Input: part model. Units: mm. Frame: model coordinates. Face numbers are marked on the shaded views. A direction names the side the tool comes from. Coordinates: 2 decimals unless noted, no trailing zeros. Write each loop counter-clockwise with the first axis right and the second up, starting at its lowest first coordinate (ties: lowest second). Pieces come first, ordered by that corner, then holes. Notation, with made-up numbers: (-7, 48) - (4, 48) arc R16 ccw to (4, 76) - close; hole circle Ø7 at (24, 87). An arc over 180 degrees is marked (long way). Use CSV: the item, a comma, the result in double quotes.
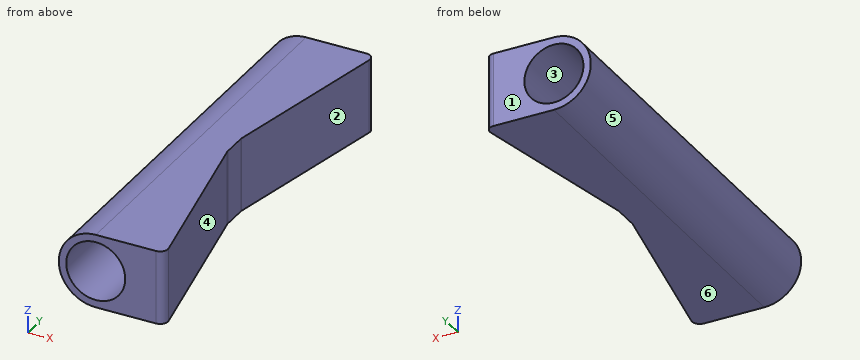
```python
from build123d import *

# Parameters (mm, degrees)
SKETCH1_R           = 14.2875
SKETCH1_R_2         = 11.4125
BOSS_EXTRUDE1_DEPTH = 152.4
SKETCH2_W           = 28.575
SKETCH2_H           = 152.4
BOSS_EXTRUDE2_DEPTH = 12.7
BOSS_EXTRUDE3_DEPTH = 152.4
CUT_EXTRUDE1_DEPTH  = 29.575
FILLET1_R           = 3


with BuildPart() as part:
    # Sketch1 → Boss-Extrude1 (new body)
    with BuildSketch(Plane(origin=(0, 0, 0), x_dir=(1, 0, 0), z_dir=(0, 1, 0))):
        Circle(SKETCH1_R)
        Circle(SKETCH1_R_2, mode=Mode.SUBTRACT)
    extrude(amount=BOSS_EXTRUDE1_DEPTH)



with BuildPart() as body_2:
    # Sketch2 → Boss-Extrude2 (new body)
    with BuildSketch(Plane(origin=(14.2875, 0, 0), x_dir=(0, 0, -1), z_dir=(1, 0, 0))):
        with Locations((0, 76.2)):
            Rectangle(SKETCH2_W, SKETCH2_H)
    extrude(amount=BOSS_EXTRUDE2_DEPTH)


with BuildPart() as part_1:
    add(part.part)

    add(body_2.part)  # Boss-Extrude3 merges body 2
    # Sketch3 → Boss-Extrude3 (add, through all)
    with BuildSketch(Plane(origin=(0, 152.4, 0), x_dir=(1, 0, 0), z_dir=(0, 1, 0))):
        with BuildLine():
            Line((14.2875, -14.2875), (0, -14.2875))
            ThreePointArc((0, -14.2875), (14.2875, 0), (0, 14.2875))
            Line((0, 14.2875), (14.2875, 14.2875))
            Line((14.2875, 14.2875), (26.9875, 14.2875))
            Line((26.9875, 14.2875), (26.9875, -14.2875))
            Line((26.9875, -14.2875), (14.2875, -14.2875))
        make_face()
    extrude(amount=-BOSS_EXTRUDE3_DEPTH)

    # Sketch5 → Cut-Extrude1 (cut, through all)
    with BuildSketch(Plane.XY.offset(14.2875)):
        Polygon((26.9875, 0), (12.897222949, 71.2), (12.897222949, 81.2), (26.9875, 152.4), align=None)
    extrude(amount=-CUT_EXTRUDE1_DEPTH, mode=Mode.SUBTRACT)

    # Fillet1
    fillet1_edges = [part_1.edges().sort_by_distance(p)[0] for p in [
        (26.9875, 0, 0),
        (26.9875, 152.4, 0),
        (12.897222949, 71.2, 0),
        (12.897222949, 81.2, 0),
    ]]
    fillet(fillet1_edges, radius=FILLET1_R)


solid = part_1.part
```
(1) Reachability of the marked faces 1 and 2 from +Z, -Z, +X, -X, +Y, -Y: full face, straight path, thin tool, end or side. Return the list, or none.
Check values:
face 1,"+Z, -Z, +X, -X, +Y"
face 2,"+Z, -Z, +X"
(2) Cut plane C-C on y = 35. Return loops of the section in (x, z) (1 decimal), and give its area (3 significant figures).
Check values:
outline,"(0, -14.3) - (20.1, -14.3) - (20.1, 14.3) - (0, 14.3) arc R14.3 ccw to start; hole circle Ø22.8 at (0, 0)"
area,"485 mm^2"
(3) Cut plane A-A on z = 0. Return loops of the section in (x, y).
Check values:
outline,"(-14.29, 0) - (-11.41, 0) - (-11.41, 152.4) - (-14.29, 152.4) - close; (11.41, 0) - (23.34, 0) arc R3 ccw to (26.28, 3.58) - (12.95, 70.91) arc R3 cw to (12.9, 71.49) - (12.9, 80.91) arc R3 cw to (12.95, 81.49) - (26.28, 148.82) arc R3 ccw to (23.34, 152.4) - (11.41, 152.4) - close"
(4) Ray query, probe 1 along X at (y, z) = (80, 0.25); probe 2 along X at (y, z) = (7, -0.25); probe 3 along Z at (x, y) = (-9, 126.5). Return the intervals inside material, ascending. Write a range as from..to.
Check values:
probe 1,"-14.29..-11.41, 11.41..12.9"
probe 2,"-14.29..-11.41, 11.41..25.6"
probe 3,"-11.1..-7.02, 7.02..11.1"
(5) Cut plane D-D on x = -8.5. Return loops of the section in (y, z), and give its area (3 significant figures).
Check values:
outline,"(0, -11.48) - (152.4, -11.48) - (152.4, -7.62) - (0, -7.62) - close; (0, 7.62) - (152.4, 7.62) - (152.4, 11.48) - (0, 11.48) - close"
area,"1,180 mm^2"
(6) Pin query (flat end, axial travel): pin 1 Ø10 at (y, z) = (74, -6) entering from +X; pin 2 Ø7.5 at (y, z) = (76.5, -5.5) entering from +X; pin 3 Ø12 at (x, z) = (-9.5, 11) entering from -Y; pin 4 Ø2 at (y, z) = (45.5, 4) entering from -X. Return the tip coordinate at first contact, or that it passes through.
Check values:
pin 1,"x = 13.33"
pin 2,"x = 12.9"
pin 3,"y = 0"
pin 4,"x = -13.97"
(7) Cut plane B-B on x = 3.5. Return loops of the section in (y, z).
Check values:
outline,"(0, -14.29) - (152.4, -14.29) - (152.4, -10.86) - (0, -10.86) - close; (0, 10.86) - (152.4, 10.86) - (152.4, 14.29) - (0, 14.29) - close"
(8) Draft query along Z for the marked faces 3, 4, 5 and 6. Return one class per face: pulls with the +Z half, pulls with the -Z half, needs draft (parallel to the pull), parting line crosses it, or undercut.
Check values:
face 3,"undercut"
face 4,"needs draft"
face 5,"parting line crosses it"
face 6,"pulls with the -Z half"
